Can you work these out from the model? Positions are in its coordinate system, mm. A direction names the side the tool comes from. Give positions to 0.01 mm unless a question says otherwise; leave off trailing zeros. Loops run counter-clockwise (first coordinate to the right, second up) from the corner with the lowest first, then second, coordinate; pieces in that order, holes last. Notation, with made-up numbers: (76, 82) - (92, 82) arc R10 cw to (92, 91) - close; hole circle Ø5 at (27, -35). An arc over 180 degrees is marked (long way). Answer as a JSON object with one key per item and string values. Group by question number.
Item 1: Suppose I cut it at B-B on z = 57. Write out the boundary of the cut face in (x, y).
Item 2: Suppose I cut it at D-D on x = -119. Write out the boundary of the cut face in (y, z).
Item 3: Which directions (+Z, -Z, +X, -X, +Y, -Y) give clear straight access to the entire face, cutting with the end or side of a thin tool? Please do faces 1 (the flat face through (-66, -27, 25.4)), 2 (the flat face through (-127, 10, 76.2)), 3 (the flat face through (-127, -53.283, 57)), 4 (the flat face through (-17, -2.483, 13)).
Item 4: Thinking about a two-plate mould opening in Y: for faces 5 (the flat face through (11.619, -66, 13)), 6 (the flat face through (-46.009, -28, 13)), 7 (the flat face through (-80, -78.683, 21)), which applies, pulls with the +Y half, pulls with the -Y half, needs draft (parallel to the pull), parting line crosses it, or undercut?
Item 5: Will these pins go through, and if not, where does the flat tip stop? pin 1 (12.5 mm diameter, centred on y = -38.5, z = 16, fed in from +X); pin 2 (5 mm diameter, centred on x = -114.5, y = -45.5, fed in from +Z); pin 3 (12 mm diameter, centred on x = -44.5, y = -36.5, fed in from +Z); pin 4 (10 mm diameter, centred on x = -4.5, y = -46, fed in from -Z).
Item 6: Suppose I cut it at C-C on z = 22. Write out the boundary of the cut face in (x, y), and give its area (3 significant figures).
Item 7: Suppose I cut it at A-A on x = -43. Write out the boundary of the cut face in (y, z).
Item 8: Please list where these lines run through material, in increasing order: L1, parallel to Y at x = -18, z = 6; L2, parallel to X at y = 15.5, z = 30.5; L3, parallel to X at y = -58, z = 13.
from build123d import *

# Parameters (mm, degrees)
F1_DEPTH = 25.4
F3_DEPTH = 25.4


with BuildPart() as f1:
    # F0 (on Top) → F1 (new body)
    with BuildSketch(Plane.XY):
        Polygon((12.468524, 22.91733), (-114.531476, 22.91733), (-114.531476, -78.68267), (11.619264, -78.68267), (11.619264, -53.28267), (-46.009442, -53.28267), (-46.009442, -2.48267), (12.468524, -2.48267), align=None)
    extrude(amount=F1_DEPTH)

    # F2 (on face) → F3 (join)
    with BuildSketch(Plane(origin=(-114.531476, 0, 0), x_dir=(0, -1, 0), z_dir=(-1, 0, 0))):
        Polygon((-22.91733, 76.2), (-22.91733, 0), (78.68267, 0), (78.68267, 76.166742), (53.28267, 76.166742), (53.28267, 36.926549), (2.48267, 36.926549), (2.48267, 76.2), align=None)
    extrude(amount=F3_DEPTH)


solid = f1.part
Worked out:
{
 "1": {"outline": "(-139.93, -78.68) - (-114.53, -78.68) - (-114.53, -53.28) - (-139.93, -53.28) - close; (-139.93, -2.48) - (-114.53, -2.48) - (-114.53, 22.92) - (-139.93, 22.92) - close"},
 "2": {"outline": "(-78.68, 0) - (22.92, 0) - (22.92, 76.2) - (-2.48, 76.2) - (-2.48, 36.93) - (-53.28, 36.93) - (-53.28, 76.17) - (-78.68, 76.17) - close"},
 "3": {"face 1": "+Z, +X, +Y, -Y", "face 2": "+Z, +X, -X, +Y, -Y", "face 3": "+Z, +X, -X", "face 4": "+Z, -Z, +X"},
 "4": {"face 5": "needs draft", "face 6": "undercut", "face 7": "pulls with the -Y half"},
 "5": {"pin 1": "stops at x = -46.01", "pin 2": "stops at z = 36.93", "pin 3": "stops at z = 25.4", "pin 4": "passes through"},
 "6": {"outline": "(-139.93, -78.68) - (11.62, -78.68) - (11.62, -53.28) - (-46.01, -53.28) - (-46.01, -2.48) - (12.47, -2.48) - (12.47, 22.92) - (-139.93, 22.92) - close", "area": "12,500 mm2"},
 "7": {"outline": "(-78.68, 0) - (-53.28, 0) - (-53.28, 25.4) - (-78.68, 25.4) - close; (-2.48, 0) - (22.92, 0) - (22.92, 25.4) - (-2.48, 25.4) - close"},
 "8": {"L1": "y = -78.68 to -53.28, -2.48 to 22.92", "L2": "x = -139.93 to -114.53", "L3": "x = -139.93 to 11.62"}
}
